from build123d import *

# Parameters (mm, degrees)
SKETCH1_R           = 7.9375
SKETCH1_R_2         = 3.175
SKETCH1_W           = 6.35
SKETCH1_H           = 38.1
BOSS_EXTRUDE1_DEPTH = 6.35
FILLET1_R           = 2.54
FILLET2_R           = 2.54


with BuildPart() as part:
    # Sketch1 → Boss-Extrude1 (new body)
    with BuildSketch(Plane.XY):
        with BuildLine():
            Line((25.4, 0), (9.525, 0))
            Line((9.525, 0), (9.525, 73.166345412))
            Line((9.525, 73.166345412), (-9.525, 73.166345412))
            Line((-9.525, 73.166345412), (-9.525, 0))
            Line((-9.525, 0), (-25.4, 0))
            Line((-25.4, 0), (-25.4, -6.35))
            Line((-25.4, -6.35), (-50.8, -6.35))
            Line((-50.8, -6.35), (-50.8, 0))
            Line((-50.8, 0), (-57.15, 0))
            Line((-57.15, 0), (-20.382757931, 231.832581844))
            ThreePointArc((-20.382757931, 231.832581844), (0, 249.2375), (20.382757931, 231.832581844))
            Line((20.382757931, 231.832581844), (57.15, 0))
            Line((57.15, 0), (50.8, 0))
            Line((50.8, 0), (50.8, -6.35))
            Line((50.8, -6.35), (25.4, -6.35))
            Line((25.4, -6.35), (25.4, 0))
        make_face()
        with Locations((0, 228.6)):
            Circle(SKETCH1_R, mode=Mode.SUBTRACT)
        with Locations((0, 242.8875)):
            Circle(SKETCH1_R_2, mode=Mode.SUBTRACT)
        with Locations((14.2875, 228.6)):
            Circle(SKETCH1_R_2, mode=Mode.SUBTRACT)
        with Locations((0, 214.3125)):
            Circle(SKETCH1_R_2, mode=Mode.SUBTRACT)
        with Locations((-14.2875, 228.6)):
            Circle(SKETCH1_R_2, mode=Mode.SUBTRACT)
        with Locations((41.275, 31.75)):
            Rectangle(SKETCH1_W, SKETCH1_H, mode=Mode.SUBTRACT)
        with Locations((-41.275, 31.75)):
            Rectangle(SKETCH1_W, SKETCH1_H, mode=Mode.SUBTRACT)
    extrude(amount=BOSS_EXTRUDE1_DEPTH)

    # Fillet1
    fillet1_edges = [part.edges().sort_by_distance(p)[0] for p in [
        (-9.525, 73.166345412, 3.175),
    ]]
    fillet(fillet1_edges, radius=FILLET1_R)

    # Fillet2
    fillet2_edges = [part.edges().sort_by_distance(p)[0] for p in [
        (9.525, 73.166345412, 3.175),
    ]]
    fillet(fillet2_edges, radius=FILLET2_R)


solid = part.part
Verification items for the finished model (mm, model axes). A direction names the side the tool comes from. Give positions to 0.01 mm unless a question says otherwise; leave off trailing zeros. Order: outer loops, then holes, each group sorted by start corner. A loop starts at its lowest first (then second) coordinate and runs counter-clockwise, first axis right, second up. Notation, with made-up numbers: M -9,58 L 1,58 A30 cw 1,96 Z; hole C 9.5,-30 d9. An arc over 180 degrees is marked long. Answer as a JSON object with one key per item and string values. Group by question number.
1) Depth check by flat-ended pin: pin 1 Ø3 at (x, z) = (2, 5.5) entering from +Y; pin 2 Ø4 at (x, y) = (0, 214.31) entering from -Z; pin 3 Ø1.9 at (x, z) = (0, 3) entering from -Y; pin 4 Ø1.9 at (y, z) = (24, 2) entering from -X. Enter the tip coordinate at first touch or a pass-through.
2) Mould release check, pull along X, two halves, no side actions. Record for faces 1 (the face through (-50.8, -3, 3)), 2 (the face through (41, 50.8, 3)), 3 (the face through (50.8, -3, 3)), 4 (the face through (18, 0, 3)): released by +X, released by -X, zero draft, split by the parting line, or undercut.
3) Cross-section at D-D (y = 62.5). Enter the section's corners in (x, z) (3 decimals).
4) Cross-section at A-A (x = 0). Enter the section's corners in (y, z).
5) Access from +Z, -Z, +X, -X, +Y, -Y to the whole of each face (thin tool, end or side, straight path). Record for faces 5 (the face through (-17, 0, 3)), 6 (the face through (38.51, 117.54, 3.13)), 7 (the face through (-54, 0, 3)), 8 (the face through (-38, -6.35, 3)), 9 (the face through (-44.45, 31, 3)).
6) Scan lines: line 1 along Y through (x, z) = (0, 4.5); line 2 along Y through (x, z) = (7, 1); line 3 along X through (y, z) = (226, 2). Record each from-to range of solid material in increasing order. Write a range as [from, to].
7) Cross-section at B-B (y = 228.6). Enter the section's corners in (x, z), then the cut area to 3 significant figures.
8) Cross-section at C-C (x = 40.5). Enter the section's corners in (y, z), then the cut area to 3 significant figures.
Result sheet:
{
 "1": {"pin 1": "stops at y = 249.23", "pin 2": "passes through", "pin 3": "stops at y = 73.17", "pin 4": "stops at x = -53.49"},
 "2": {"face 1": "released by -X", "face 2": "undercut", "face 3": "released by +X", "face 4": "undercut"},
 "3": {"outline": "M -47.238,0 L -9.525,0 L -9.525,6.35 L -47.238,6.35 Z; M 9.525,0 L 47.238,0 L 47.238,6.35 L 9.525,6.35 Z"},
 "4": {"outline": "M 73.17,0 L 211.14,0 L 211.14,6.35 L 73.17,6.35 Z; M 217.49,0 L 220.66,0 L 220.66,6.35 L 217.49,6.35 Z; M 236.54,0 L 239.71,0 L 239.71,6.35 L 236.54,6.35 Z; M 246.06,0 L 249.24,0 L 249.24,6.35 L 246.06,6.35 Z"},
 "5": {"face 5": "+Z, -Z, -Y", "face 6": "+Z, -Z, +X, +Y", "face 7": "+Z, -Z, -X, -Y", "face 8": "+Z, -Z, +X, -X, -Y", "face 9": "+Z, -Z"},
 "6": {"line 1": "y = [73.17, 211.14], [217.49, 220.66], [236.54, 239.71], [246.06, 249.24]", "line 2": "y = [73.17, 224.86], [232.34, 248.01]", "line 3": "x = [-21.31, -16.11], [-12.47, -7.5], [7.5, 12.47], [16.11, 21.31]"},
 "7": {"outline": "M -20.9,0 L -17.46,0 L -17.46,6.35 L -20.9,6.35 Z; M -11.11,0 L -7.94,0 L -7.94,6.35 L -11.11,6.35 Z; M 7.94,0 L 11.11,0 L 11.11,6.35 L 7.94,6.35 Z; M 17.46,0 L 20.9,0 L 20.9,6.35 L 17.46,6.35 Z", "area": "83.9 mm2"},
 "8": {"outline": "M -6.35,0 L 12.7,0 L 12.7,6.35 L -6.35,6.35 Z; M 50.8,0 L 104.99,0 L 104.99,6.35 L 50.8,6.35 Z", "area": "465 mm2"}
}
